Build history of the part. All positions in model axes, mm. A direction names the side the tool comes from. Coordinates: 2 decimals unless noted, no trailing zeros. Write each loop counter-clockwise with the first axis right and the second up, starting at its lowest first coordinate (ties: lowest second). Pieces come first, ordered by that corner, then holes.
```python
from build123d import *

# Parameters (mm, degrees)
EXTRUDE_1_DEPTH      = 8
FILLET_1_R           = 3
SKETCH_3_R           = 2
CUT_EXTRUDE_1_DEPTH  = 60
SKETCH_4_R           = 2
CUT_EXTRUDE_2_DEPTH  = 50
MIRROR_1_OUTLINE_R   = 2
MIRROR_1_DEPTH       = 1.9999999
MIRROR_START         = 6.0000001
MIRROR_1_2_OUTLINE_R = 2
MIRROR_1_2_DEPTH     = 1.9999999
MIRROR_START_2       = 1.9999999
MIRROR_1_3_OUTLINE_R = 2
MIRROR_1_3_DEPTH     = 4.0000002
MIRROR_START_3       = -1
MIRROR_1_4_OUTLINE_R = 2
MIRROR_1_4_DEPTH     = 61
SKETCH_5_R           = 2
CUT_EXTRUDE_3_DEPTH  = 100


with BuildPart() as part:
    # 草图1 → 凸台-拉伸1 (new body)
    with BuildSketch(Plane.XY):
        Polygon((0, 0), (32, 0), (32, 10), (22, 10), (22, 48.6), (32, 48.6), (32, 58.6), (0, 58.6), (0, 48.6), (10, 48.6), (10, 10), (0, 10), align=None)
    extrude(amount=EXTRUDE_1_DEPTH)

    # 圆角1
    fillet_1_edges = [part.edges().sort_by_distance(p)[0] for p in [
        (10, 10, 4),
        (10, 48.6, 4),
        (22, 48.6, 4),
        (22, 10, 4),
    ]]
    fillet(fillet_1_edges, radius=FILLET_1_R)

    # 草图3 → 切除-拉伸1 (cut)
    with BuildSketch(Plane(origin=(0, 58.6, 0), x_dir=(1, 0, 0), z_dir=(0, 1, 0))):
        with Locations(Location((4, -4, 0), (0, 0, 270))):
            Circle(SKETCH_3_R)
    extrude(amount=-CUT_EXTRUDE_1_DEPTH, mode=Mode.SUBTRACT)

    # 草图4 → 切除-拉伸2 (cut)
    with BuildSketch(Plane.XY.offset(8)):
        with Locations((16, 53.6)):
            Circle(SKETCH_4_R)
        with Locations(Location((16, 5, 0), (0, 0, 180))):
            Circle(SKETCH_4_R)
    extrude(amount=-CUT_EXTRUDE_2_DEPTH, mode=Mode.SUBTRACT)

    # 镜向1: read off the stored shape, not the designer's step
    # 镜向1 outline → 镜向1 (add)
    with BuildSketch(Plane.XY):
        with BuildLine():
            Line((32, 0), (64, 0))
            Line((64, 0), (64, 10))
            Line((64, 10), (57, 10))
            ThreePointArc((57, 10), (54.878679656, 10.878679656), (54, 13))
            Line((54, 13), (54, 45.6))
            ThreePointArc((54, 45.6), (54.878679656, 47.721320344), (57, 48.6))
            Line((57, 48.6), (64, 48.6))
            Line((64, 48.6), (64, 58.6))
            Line((64, 58.6), (32, 58.6))
            Line((32, 58.6), (32, 48.6))
            Line((32, 48.6), (39, 48.6))
            ThreePointArc((39, 48.6), (41.121320344, 47.721320344), (42, 45.6))
            Line((42, 45.6), (42, 13))
            ThreePointArc((42, 13), (41.121320344, 10.878679656), (39, 10))
            Line((39, 10), (32, 10))
            Line((32, 10), (32, 0))
        make_face()
        with Locations((48, 5)):
            Circle(MIRROR_1_OUTLINE_R, mode=Mode.SUBTRACT)
        with Locations((48, 53.6)):
            Circle(MIRROR_1_OUTLINE_R, mode=Mode.SUBTRACT)
    extrude(amount=MIRROR_1_DEPTH)

    # Mirror 1 2 outline → Mirror 1 2 (add)
    with BuildSketch(Plane.XY.offset(MIRROR_START)):
        with BuildLine():
            Line((32, 0), (64, 0))
            Line((64, 0), (64, 10))
            Line((64, 10), (57, 10))
            ThreePointArc((57, 10), (54.878679656, 10.878679656), (54, 13))
            Line((54, 13), (54, 45.6))
            ThreePointArc((54, 45.6), (54.878679656, 47.721320344), (57, 48.6))
            Line((57, 48.6), (64, 48.6))
            Line((64, 48.6), (64, 58.6))
            Line((64, 58.6), (32, 58.6))
            Line((32, 58.6), (32, 48.6))
            Line((32, 48.6), (39, 48.6))
            ThreePointArc((39, 48.6), (41.121320344, 47.721320344), (42, 45.6))
            Line((42, 45.6), (42, 13))
            ThreePointArc((42, 13), (41.121320344, 10.878679656), (39, 10))
            Line((39, 10), (32, 10))
            Line((32, 10), (32, 0))
        make_face()
        with Locations((48, 5)):
            Circle(MIRROR_1_2_OUTLINE_R, mode=Mode.SUBTRACT)
        with Locations((48, 53.6)):
            Circle(MIRROR_1_2_OUTLINE_R, mode=Mode.SUBTRACT)
    extrude(amount=MIRROR_1_2_DEPTH)

    # Mirror 1 3 outline → Mirror 1 3 (add)
    with BuildSketch(Plane.XY.offset(MIRROR_START_2)):
        with BuildLine():
            Line((32, 0), (64, 0))
            Line((64, 0), (64, 10))
            Line((64, 10), (57, 10))
            ThreePointArc((57, 10), (54.878679656, 10.878679656), (54, 13))
            Line((54, 13), (54, 45.6))
            ThreePointArc((54, 45.6), (54.878679656, 47.721320344), (57, 48.6))
            Line((57, 48.6), (64, 48.6))
            Line((64, 48.6), (64, 58.6))
            Line((64, 58.6), (32, 58.6))
            Line((32, 58.6), (32, 48.6))
            Line((32, 48.6), (39, 48.6))
            ThreePointArc((39, 48.6), (41.121320344, 47.721320344), (42, 45.6))
            Line((42, 45.6), (42, 13))
            ThreePointArc((42, 13), (41.121320344, 10.878679656), (39, 10))
            Line((39, 10), (32, 10))
            Line((32, 10), (32, 0))
        make_face()
        with Locations((48, 5)):
            Circle(MIRROR_1_3_OUTLINE_R, mode=Mode.SUBTRACT)
        with Locations((48, 53.6)):
            Circle(MIRROR_1_3_OUTLINE_R, mode=Mode.SUBTRACT)
    extrude(amount=MIRROR_1_3_DEPTH)

    # Mirror 1 4 outline → Mirror 1 4 (cut)
    with BuildSketch(Plane(origin=(0, 0, 0), x_dir=(1, 0, 0), z_dir=(0, 1, 0)).offset(MIRROR_START_3)):
        with Locations((60, -4)):
            Circle(MIRROR_1_4_OUTLINE_R)
    extrude(amount=MIRROR_1_4_DEPTH, mode=Mode.SUBTRACT)

    # 草图5 → 切除-拉伸3 (cut)
    with BuildSketch(Plane.XZ):
        with Locations(Location((32, 4, 0), (0, 0, 270))):
            Circle(SKETCH_5_R)
    extrude(amount=-CUT_EXTRUDE_3_DEPTH, mode=Mode.SUBTRACT)


solid = part.part
```
1. Saw through at A-A on y = 53.6. List the corners of the cut face in (x, z), plus the area to 3 significant figures.
Computed values:
outline: (0, 0) - (14, 0) - (14, 8) - (0, 8) - close; (18, 0) - (46, 0) - (46, 8) - (18, 8) - close; (50, 0) - (64, 0) - (64, 8) - (50, 8) - close; hole circle Ø4 at (4, 4); hole circle Ø4 at (32, 4); hole circle Ø4 at (60, 4)
area: 410 mm2
2. Saw through at C-C on y = 21.5. List the corners of the cut face in (x, z), plus the area to 3 significant figures.
Computed values:
outline: (10, 0) - (22, 0) - (22, 8) - (10, 8) - close; (42, 0) - (54, 0) - (54, 8) - (42, 8) - close
area: 192 mm2
3. 3-axis set-ups, long thin cutter, end or side, ignore diameter. For faces 1 (the face through (22.9, 10.86, 4.06)), 2 (the face through (54, 29, 4)), 3 (the face through (10, 30, 4)): which of +Z, -Z, +X, -X, +Y, -Y reach the whole face in a straight line?
Computed values:
face 1: +Z, -Z
face 2: +Z, -Z, +X
face 3: +Z, -Z, -X
4. Flat gauge pin, fed straight in: pin 1 (2.5 mm diameter, centred on y = 33, z = 2, fed in from -X). Where does the tip first touch, or does it go through?
Computed values:
pin 1: stops at x = 10
5. Saw through at B-B on x = 48. List the corners of the cut face in (y, z).
Computed values:
outline: (0, 0) - (3, 0) - (3, 8) - (0, 8) - close; (7, 0) - (51.6, 0) - (51.6, 8) - (7, 8) - close; (55.6, 0) - (58.6, 0) - (58.6, 8) - (55.6, 8) - close
6. Probe line 1 along Y through (x, z) = (16, 4.25); line 2 along X through (y, z) = (24, 2); line 3 along Y through (x, z) = (3.5, 6.5). List the from-to ranges inside material, lowest first.
Computed values:
line 1: y = 0 to 3, 7 to 51.6, 55.6 to 58.6
line 2: x = 10 to 22, 42 to 54
line 3: y = 0 to 10, 48.6 to 58.6
7. Mould opens along X. For faces 4 (the face through (9.14, 10.9, 4.06)), 5 (the face through (34, 10, 6)), 6 (the face through (32, 58.6, 1)) say: +X half, -X half, draft (parallel to the pull), parting line (faces both ways), or undercut.
Computed values:
face 4: -X half
face 5: undercut
face 6: draft
8. Saw through at D-D on z = 6.75. List the corners of the cut face in (x, y).
Computed values:
outline: (0, 0) - (64, 0) - (64, 10) - (57, 10) arc R3 cw to (54, 13) - (54, 45.6) arc R3 cw to (57, 48.6) - (64, 48.6) - (64, 58.6) - (0, 58.6) - (0, 48.6) - (7, 48.6) arc R3 cw to (10, 45.6) - (10, 13) arc R3 cw to (7, 10) - (0, 10) - close; hole circle Ø4 at (16, 5); hole circle Ø4 at (16, 53.6); hole (22, 13) arc R3 ccw to (25, 10) - (39, 10) arc R3 ccw to (42, 13) - (42, 45.6) arc R3 ccw to (39, 48.6) - (25, 48.6) arc R3 ccw to (22, 45.6) - close; hole circle Ø4 at (48, 5); hole circle Ø4 at (48, 53.6)
